Geometry: final body of the model. Coordinates: model frame, mm. A direction names the side the tool comes from. Round coordinates to 2 decimals unless told otherwise and drop trailing zeros. Order: outer loops, then holes, each group sorted by start corner. A loop starts at its lowest first (then second) coordinate and runs counter-clockwise, first axis right, second up. Notation, with made-up numbers: (-33, 86) -> (10, 86) arc R19 cw to (10, 115) -> close; hole circle Ø4 at (31, 38). An arc over 180 degrees is marked (long way). Put each result on its own line as item: value.
```python
from build123d import *

# Parameters (mm, degrees)
F0_R           = 53.975
F1_DEPTH       = 63.5
F3_D           = 16.66748
F3_CBORE_D     = 25.4
F3_CBORE_DEPTH = 31.75
F4_SIZE        = 6.35


with BuildPart() as f1:
    # F0 (on Top) → F1 (new body)
    with BuildSketch(Plane.XY):
        Circle(F0_R)
    extrude(amount=F1_DEPTH)

    # F3 (through all)
    with Locations(Plane.XY.offset(63.5)):
        with Locations((0, 0)):
            CounterBoreHole(F3_D / 2, F3_CBORE_D / 2, F3_CBORE_DEPTH)

    # F4
    f4_edges = [f1.edges().sort_by_distance(p)[0] for p in [
        (-53.975, 0, 0),
    ]]
    chamfer(f4_edges, length=F4_SIZE)


solid = f1.part
```
1. Cut plane A-A on y = 0. Return loops of the section in (x, z) (3 decimals), and give its area (3 significant figures).
Ans:
outline: (-53.975, 6.35) -> (-47.625, 0) -> (-8.334, 0) -> (-8.334, 31.75) -> (-12.7, 31.75) -> (-12.7, 63.5) -> (-53.975, 63.5) -> close; (8.334, 0) -> (47.625, 0) -> (53.975, 6.35) -> (53.975, 63.5) -> (12.7, 63.5) -> (12.7, 31.75) -> (8.334, 31.75) -> close
area: 5,480 mm²
2. Material intervals for probe 1 along Y at (x, z) = (0, 23) (3 decimals); probe 2 along Y at (x, z) = (0, 51) (3 decimals); probe 3 along Z at (x, y) = (8.5, -9), sorted ascending.
Ans:
probe 1: -53.975 to -8.334, 8.334 to 53.975
probe 2: -53.975 to -12.7, 12.7 to 53.975
probe 3: 0 to 31.75
3. Draft query along X for faces 1 (the face through (8.326, 0.366, 15.653)), 2 (the face through (-39.78, 36.48, 34.52)), 3 (the face through (-1, -10, 0)). Return one class per face: +X half, -X half, draft (parallel to the pull), parting line (faces both ways), or undercut.
Ans:
face 1: undercut
face 2: parting line
face 3: draft
4. Set-up query: faces 4 (the face through (45.72, 14.4, 0.31)), 5 (the face through (3, -8, 31.75)). Return all of +Z, -Z, +X, -X, +Y, -Y with unobstructed straight access to the full face (end or side cutting, diameter ignored); none if empty.
Ans:
face 4: -Z
face 5: +Z
5. Contact query for flat-ended pins moving along their axis: P1, Ø1.5, axis at x = 15.5, z = 51, coming from the +Y side; P2, Ø21.5, axis at x = 0, y = 0, coming from the +Z side; P3, Ø10, axis at y = 13.5, z = 56, coming from the -X side. Output: stop coordinate, or through.
Ans:
P1: y = 51.92
P2: z = 31.75
P3: x = -53.3
6. Cut plane C-C on z = 36. Return loops of the section in (x, y) (3 decimals).
Ans:
outline: circle Ø107.95 at (0, 0); hole circle Ø25.4 at (0, 0)
7. Cut plane D-D on z = 8.5. Return loops of the section in (x, y) (3 decimals), and give its area (3 significant figures).
Ans:
outline: circle Ø107.95 at (0, 0); hole circle Ø16.667 at (0, 0)
area: 8,930 mm²
